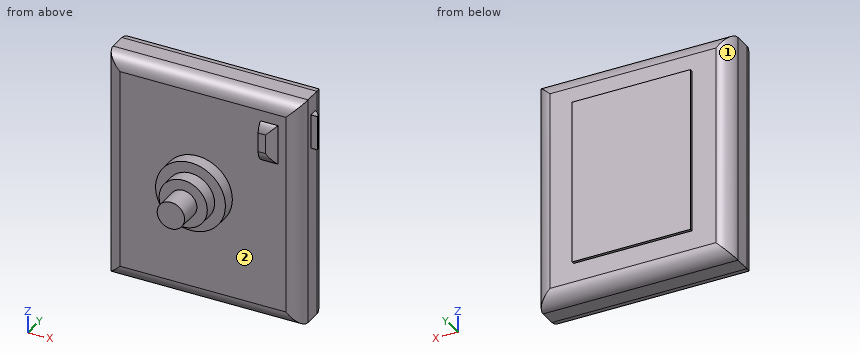
```python
from build123d import *

# Parameters (mm, degrees)
F0_W         = 68.5527212918
F0_H         = 80.7738155127
F1_DEPTH     = 16.002
F2_R         = 12.2829248395
F2_W         = 6.1860904098
F2_H         = 13.9971412718
F4_DEPTH     = 1.524
F5_DEPTH     = 3.048
F3_W         = 2.9572332278
F3_H         = 12.0760332793
F6_DEPTH     = 2.54
F7_T1_DEPTH  = 34.0730785354
F8_R         = 8.4752207388
F9_DEPTH     = 4.826
F10_R        = 4.8104699567
F11_DEPTH    = 8.128
F12_R        = 5.08
F13_T1_DEPTH = 32.1363694803
F13_T3_DEPTH = 24.3253186183
F14_W        = 41.5736716241
F14_H        = 57.9494982958
F15_DEPTH    = 1.016


# Not quite as in the source:
# - a fillet or chamfer that OpenCascade refuses, or shapes differently, is made with other operations: its cross-section is extruded or revolved along the edge and cut away or added


with BuildPart() as f1:
    # F0 (on Front) → F1 (new body)
    with BuildSketch(Plane.XZ):
        with Locations((1.9095446914, -0.1909546554)):
            Rectangle(F0_W, F0_H)
    extrude(amount=F1_DEPTH)

    # F2 (on face) → F4 (join)
    with BuildSketch(Plane.XZ.offset(16.002)):
        Circle(F2_R)
        with Locations((25.2598635852, 24.3296492845)):
            Rectangle(F2_W, F2_H)
    extrude(amount=F4_DEPTH)

    # F5 (add): a face of the model
    f5_faces = [f1.faces().sort_by_distance(p)[0] for p in [
        (0, -17.526, 0),
    ]]
    extrude(f5_faces, amount=F5_DEPTH)

    # F3 (on face) → F6 (join)
    with BuildSketch(Plane.YZ.offset(36.1859053373)):
        with Locations((-7.535086479, 27.7017401531)):
            Rectangle(F3_W, F3_H)
    extrude(amount=F6_DEPTH)

    # F7: fillet of radius 5.08 on 1 edges, made by hand

    # F7_s2 → F7_t1 (cut)
    with BuildSketch(Plane.XY.offset(10.6652008854)):
        with BuildLine():
            ThreePointArc((36.1859053373, -6.0564698651), (38.0453143886, -7.9158789164), (38.7259053373, -10.4558789164))
            Line((38.7259053373, -10.4558789164), (38.7259053373, -6.0564698651))
            Line((38.7259053373, -6.0564698651), (36.1859053373, -6.0564698651))
        make_face()
    extrude(amount=F7_T1_DEPTH, mode=Mode.SUBTRACT)

    # F8 (on face) → F9 (join)
    with BuildSketch(Plane.XZ.offset(20.574)):
        Circle(F8_R)
    extrude(amount=F9_DEPTH)

    # F10 (on face) → F11 (join)
    with BuildSketch(Plane.XZ.offset(25.4)):
        Circle(F10_R)
    extrude(amount=F11_DEPTH)

    # F12
    f12_edges = [f1.edges().sort_by_distance(p)[0] for p in [
        (36.185905, -16.002, -0.190955),
        (1.909545, -16.002, 40.195953),
        (1.909545, -16.002, -40.577862),
        (-32.366816, -16.002, -0.190955),
        (1.909545, 0, -40.577862),
        (36.185905, 0, -0.190955),
        (1.909545, 0, 40.195953),
        (-32.366816, 0, -0.190955),
    ]]
    fillet(f12_edges, radius=F12_R)

    # F13: fillet of radius 5.08 on 3 edges, made by hand

    # F13_s2 → F13_t1 (cut)
    with BuildSketch(Plane.XY.offset(8.2614645443)):
        with BuildLine():
            ThreePointArc((28.3529087901, -16.002), (26.6925386883, -17.1295285843), (24.7250631484, -17.526))
            Line((24.7250631484, -17.526), (28.3529087901, -17.526))
            Line((28.3529087901, -17.526), (28.3529087901, -16.002))
        make_face()
    extrude(amount=F13_T1_DEPTH, mode=Mode.SUBTRACT)

    # F13_s4 → F13_t3 (cut)
    with BuildSketch(Plane.YZ.offset(13.0972042761)):
        with BuildLine():
            ThreePointArc((-16.002, 31.3282199204), (-17.1295285843, 29.6678498186), (-17.526, 27.7003742787))
            Line((-17.526, 27.7003742787), (-17.526, 31.3282199204))
            Line((-17.526, 31.3282199204), (-16.002, 31.3282199204))
        make_face()
        with BuildLine():
            ThreePointArc((-16.002, 17.3310786486), (-17.1295285843, 18.9914487504), (-17.526, 20.9589242903))
            Line((-17.526, 20.9589242903), (-17.526, 17.3310786486))
            Line((-17.526, 17.3310786486), (-16.002, 17.3310786486))
        make_face()
    extrude(amount=F13_T3_DEPTH, mode=Mode.SUBTRACT)

    # F14 (on face) → F15 (join)
    with BuildSketch(Plane(origin=(0, 0, 0), x_dir=(-1, 0, 0), z_dir=(0, 1, 0))):
        with Locations((-1.9210586324, 0.1702420413)):
            Rectangle(F14_W, F14_H)
    extrude(amount=F15_DEPTH)


solid = f1.part
```
Geometry: final body of the model. Coordinates: model frame, mm. Face numbers are marked on the shaded views. A direction names the side the tool comes from. Round coordinates to 2 decimals unless told otherwise and drop trailing zeros. Order: outer loops, then holes, each group sorted by start corner. A loop starts at its lowest first (then second) coordinate and runs counter-clockwise, first axis right, second up. Notation, with made-up numbers: (64.25, -23.75) -> (92.25, -23.75) arc R34 cw to (92.25, 11.25) -> close; hole circle Ø10 at (62, 28). An arc over 180 degrees is marked (long way). Use one line per item in the form item = value. Start each with the question number.
1. Cut plane B-B (x = 0). Return the cut outline in (y, z) (1 decimal).
2. Cut plane D-D (z = 16). Return the cut outline in (x, y), then the cut area to 3 significant figures.
3. Reachability of the marked faces 1 and 2 from +Z, -Z, +X, -X, +Y, -Y: full face, straight path, thin tool, end or side. Return the list, or none.
4. Cut plane C-C (y = -29). Return the cut outline in (x, z), then the cut area to 3 significant figures.
5. Cut plane A-A (z = 0). Return the cut outline in (x, y).
6. Line query: probe 1 along Y at (x, z) = (8, -8); probe 2 along Y at (x, z) = (24.5, -24); probe 3 along Z at (x, y) = (-6, -20). Output: solid intervals per line, ascending.
7. Pin query (flat end, axial travel): pin 1 Ø1.2 at (x, y) = (37, -7.5) entering from +Z; pin 2 Ø12 at (y, z) = (-22.5, -31.5) entering from +X; pin 3 Ø2 at (y, z) = (-9, -25.5) entering from +X; pin 4 Ø0.5 at (x, y) = (-2.5, 0.5) entering from -Z. Return the tip coordinate at first contact, or that it passes through.
Solution:
q1.outline = (-33.5, -4.8) -> (-25.4, -4.8) -> (-25.4, -8.5) -> (-20.6, -8.5) -> (-20.6, -12.3) -> (-16, -12.3) -> (-16, -35.5) arc R5.1 ccw to (-10.9, -40.6) -> (-5.1, -40.6) arc R5.1 ccw to (0, -35.5) -> (0, -28.8) -> (1, -28.8) -> (1, 29.1) -> (0, 29.1) -> (0, 35.1) arc R5.1 ccw to (-5.1, 40.2) -> (-10.9, 40.2) arc R5.1 ccw to (-16, 35.1) -> (-16, 12.3) -> (-20.6, 12.3) -> (-20.6, 8.5) -> (-25.4, 8.5) -> (-25.4, 4.8) -> (-33.5, 4.8) -> close
q2.outline = (-32.37, -10.92) arc R5.08 ccw to (-27.29, -16) -> (31.11, -16) arc R5.08 ccw to (36.19, -10.92) -> (36.19, -5.08) arc R5.08 ccw to (31.11, 0) -> (22.71, 0) -> (22.71, 1.02) -> (-18.87, 1.02) -> (-18.87, 0) -> (-27.29, 0) arc R5.08 ccw to (-32.37, -5.08) -> close
q2.area = 1,120 mm^2
q3.face_1 = +Z, -Z, -X, +Y
q3.face_2 = -Y
q4.outline = circle Ø9.62 at (0, 0)
q4.area = 72.7 mm^2
q5.outline = (-32.37, -10.92) arc R5.08 ccw to (-27.29, -16) -> (-12.28, -16) -> (-12.28, -20.57) -> (-8.48, -20.57) -> (-8.48, -25.4) -> (-4.81, -25.4) -> (-4.81, -33.53) -> (4.81, -33.53) -> (4.81, -25.4) -> (8.48, -25.4) -> (8.48, -20.57) -> (12.28, -20.57) -> (12.28, -16) -> (31.11, -16) arc R5.08 ccw to (36.19, -10.92) -> (36.19, -5.08) arc R5.08 ccw to (31.11, 0) -> (22.71, 0) -> (22.71, 1.02) -> (-18.87, 1.02) -> (-18.87, 0) -> (-27.29, 0) arc R5.08 ccw to (-32.37, -5.08) -> close
q6.probe_1 = -20.57 to 1.02
q6.probe_2 = -16 to 0
q6.probe_3 = -10.72 to 10.72
q7.pin_1 = 33.74
q7.pin_2 = through
q7.pin_3 = 36.19
q7.pin_4 = -28.8
